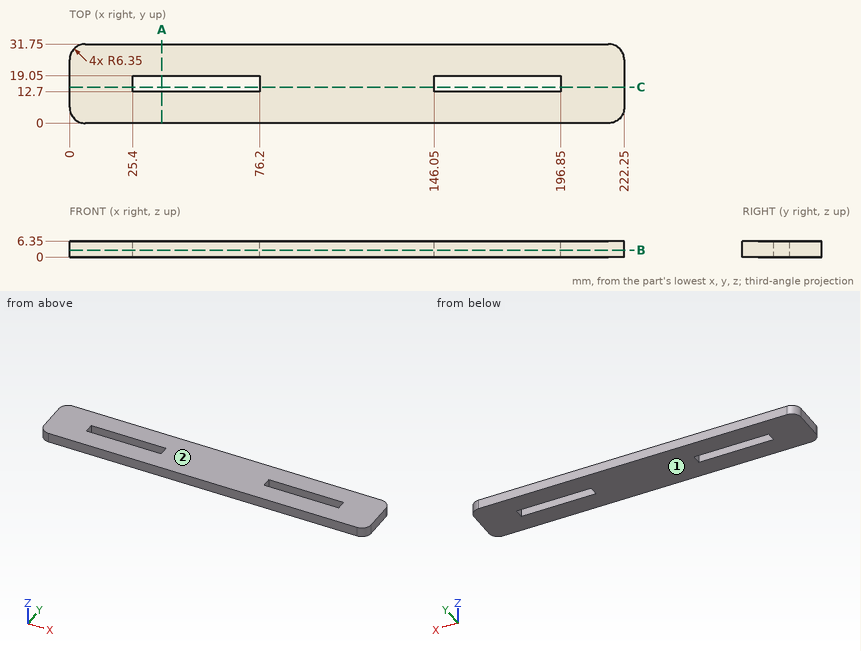
Can you work these out from the drawing? Everything is in mm from the part's minimum corner. Give positions to 0.01 mm unless a question says otherwise; leave off trailing zeros. Loops run counter-clockwise (first coordinate to the right, second up) from the corner with the lowest first, then second, coordinate; pieces in that order, holes last. Notation, with made-up numbers: (67, -20.5) -> (109, -20.5) arc R32 cw to (109, 15.5) -> close; hole circle Ø4 at (40.25, 11.25). An arc over 180 degrees is marked (long way). Put each result on its own line as item: value.
(1) Thinking about a two-plate mould opening in Z: for the marked faces 1 and 2, which applies, pulls with the +Z half, pulls with the -Z half, needs draft (parallel to the pull), parting line crosses it, or undercut?
Computed:
face 1: pulls with the -Z half
face 2: pulls with the +Z half
(2) Please list where these lines run through material, in increasing order: probe 1 along X at (y, z) = (17.5, 3.75); probe 2 along Y at (x, z) = (55, 2.5); probe 3 along X at (y, z) = (6, 2.5). Write a range as [from, to].
Computed:
probe 1: [0, 25.4], [76.2, 146.05], [196.85, 222.25]
probe 2: [0, 12.7], [19.05, 31.75]
probe 3: [0.01, 222.24]
(3) Imagine slicing it at B-B on z = 2.75. Write out the boundary of the cut face in (x, y).
Computed:
outline: (0, 6.35) arc R6.35 ccw to (6.35, 0) -> (215.9, 0) arc R6.35 ccw to (222.25, 6.35) -> (222.25, 25.4) arc R6.35 ccw to (215.9, 31.75) -> (6.35, 31.75) arc R6.35 ccw to (0, 25.4) -> close; hole (25.4, 12.7) -> (76.2, 12.7) -> (76.2, 19.05) -> (25.4, 19.05) -> close; hole (146.05, 12.7) -> (196.85, 12.7) -> (196.85, 19.05) -> (146.05, 19.05) -> close
(4) Imagine slicing it at A-A on x = 37. Write out the boundary of the cut face in (y, z).
Computed:
outline: (0, 0) -> (12.7, 0) -> (12.7, 6.35) -> (0, 6.35) -> close; (19.05, 0) -> (31.75, 0) -> (31.75, 6.35) -> (19.05, 6.35) -> close
(5) Imagine slicing it at C-C on y = 14.5. Write out the boundary of the cut face in (x, z), plus the area to 3 significant figures.
Computed:
outline: (0, 0) -> (25.4, 0) -> (25.4, 6.35) -> (0, 6.35) -> close; (76.2, 0) -> (146.05, 0) -> (146.05, 6.35) -> (76.2, 6.35) -> close; (196.85, 0) -> (222.25, 0) -> (222.25, 6.35) -> (196.85, 6.35) -> close
area: 766 mm^2
